Could you check a few things on this model? Use its own coordinates, in mm. Face numbers are marked on the shaded views. A direction names the side the tool comes from. Give positions to 0.01 mm unless a question says otherwise; leave off trailing zeros. Loops run counter-clockwise (first coordinate to the right, second up) from the corner with the lowest first, then second, coordinate; pieces in that order, holes last. Notation, with made-up numbers: (60, 72) - (102, 72) arc R14 ccw to (102, 86) - close; hole circle Ø1 at (72.5, 88). An arc over 180 degrees is marked (long way). One line per item, written item: value. Start each with the question number.
Q1. I want a section at D-D (z = -25). Please give me the cut outline in (x, y).
Q2. I want a section at C-C (z = 54.5). Please give me the cut outline in (x, y).
Q3. I want a section at A-A (z = 0). Please give me the cut outline in (x, y), then the cut area to 3 significant figures.
Q4. I want a section at B-B (y = -16). Please give me the cut outline in (x, z), then the cut area to 3 significant figures.
Q5. If I drill on line 1 (Y direction, x = 12, z = -1); line 2 (Y direction, x = 4, z = 43); line 3 (Z direction, x = -0.5, y = -39.5), over which ranges is the centre line in solid material (lowest first)? Write a range as from..to.
Q6. I'm going to push flat-ended pins straight in: P1, Ø1, axis at y = -1, z = -20.5, coming from the +X side; P2, Ø8, axis at x = 25.5, z = -15, coming from the -Y side; P3, Ø2, axis at x = 10, y = -43, coming from the +Z side; P4, Ø5, axis at x = 8, z = -6.5, coming from the +Y side. Where does each tip first touch, or does it pass through?
Q7. For the marked faces 5 and 6, which set-ups out of +Z, -Z, +X, -X, +Y, -Y let a thin tool reach every point of the face, with its end or its side?
Q8. If we mould it in two halves opening along Z, with no side actions, what happens to the marked faces 1, 2, 3 and 4? For each: released by +Z, released by -Z, zero draft, split by the parting line, or undercut.
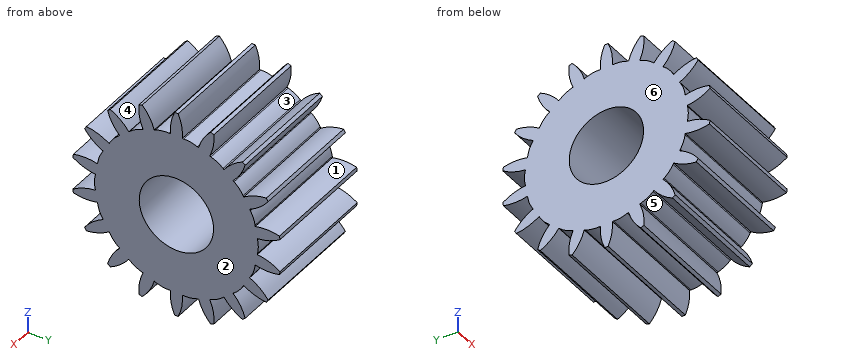
```python
from build123d import *

# Parameters (mm, degrees)
SKETCH1_R                = 63.5
BOSS_EXTRUDE1_DEPTH      = 35
SKETCH6_R                = 22.5
CUT_EXTRUDE4_DEPTH       = 71
CUT_EXTRUDE5_DEPTH       = 71
FILLET1_R                = 20
CIRPATTERN3_COUNT        = 18
FILLET1_OF_CIRPATTERN3_R = 20


with BuildPart() as part:
    # Sketch1 → Boss-Extrude1 (new body, symmetric)
    with BuildSketch(Plane(origin=(0, 0, 0), x_dir=(0, 0, -1), z_dir=(1, 0, 0))):
        Circle(SKETCH1_R)
    extrude(amount=BOSS_EXTRUDE1_DEPTH, both=True)

    # Sketch6 → Cut-Extrude4 (cut, through all)
    with BuildSketch(Plane(origin=(35, 0, 0), x_dir=(0, 0, -1), z_dir=(1, 0, 0))):
        Circle(SKETCH6_R)
    extrude(amount=-CUT_EXTRUDE4_DEPTH, mode=Mode.SUBTRACT)

    # Sketch7 → Cut-Extrude5 (cut, through all)
    with BuildSketch(Plane(origin=(35, 0, 0), x_dir=(0, 0, -1), z_dir=(1, 0, 0))):
        with BuildLine():
            Line((0, 50.039601818), (-4.985, 48.961883134))
            ThreePointArc((-4.985, 48.961883134), (-6.597219376, 56.157134763), (-9.975, 62.711636679))
            Line((-9.975, 62.711636679), (0, 72.167588378))
            Line((0, 72.167588378), (9.975, 62.711636679))
            ThreePointArc((9.975, 62.711636679), (6.597219376, 56.157134763), (4.985, 48.961883134))
            Line((4.985, 48.961883134), (0, 50.039601818))
        make_face()
    cut_extrude5 = extrude(amount=-CUT_EXTRUDE5_DEPTH, mode=Mode.SUBTRACT)

    # Fillet1
    fillet1_edges = [part.edges().sort_by_distance(p)[0] for p in [
        (0, 50.039601818, 0),
    ]]
    fillet(fillet1_edges, radius=FILLET1_R)

    # CirPattern3: Cut-Extrude5 ×18 about axis
    cirpattern3_axis = Axis((0, 0, 0), (1, 0, 0))
    for i in range(1, CIRPATTERN3_COUNT):
        add(cut_extrude5.rotate(cirpattern3_axis, i * 360 / CIRPATTERN3_COUNT), mode=Mode.SUBTRACT)

    # Fillet1 of CirPattern3
    fillet1_of_cirpattern3_edges = [part.edges().sort_by_distance(p)[0] for p in [
        (0, 47.021844575, 17.114551786),
        (0, 38.332558908, 32.164836042),
        (0, 25.019800909, 43.335566369),
        (0, 8.689285667, 49.279387828),
        (0, -8.689285667, 49.279387828),
        (0, -25.019800909, 43.335566369),
        (0, -38.332558908, 32.164836042),
        (0, -47.021844575, 17.114551786),
        (0, -50.039601818, 0),
        (0, -47.021844575, -17.114551786),
        (0, -38.332558908, -32.164836042),
        (0, -25.019800909, -43.335566369),
        (0, -8.689285667, -49.279387828),
        (0, 8.689285667, -49.279387828),
        (0, 25.019800909, -43.335566369),
        (0, 38.332558908, -32.164836042),
        (0, 47.021844575, -17.114551786),
    ]]
    fillet(fillet1_of_cirpattern3_edges, radius=FILLET1_OF_CIRPATTERN3_R)


solid = part.part
```
Worked answers:
1. outline: (-35, -50.02) - (35, -50.02) - (35, 50.02) - (-35, 50.02) - close
2. outline: (-35, -22.7) - (35, -22.7) - (35, -16.45) - (-35, -16.45) - close; (-35, -3.53) - (35, -3.53) - (35, 3.53) - (-35, 3.53) - close; (-35, 16.45) - (35, 16.45) - (35, 22.7) - (-35, 22.7) - close
3. outline: (-35, -49.58) - (35, -49.58) - (35, -22.5) - (-35, -22.5) - close; (-35, 22.5) - (35, 22.5) - (35, 49.58) - (-35, 49.58) - close
3. area: 3,790 mm²
4. outline: (-35, -53.72) - (35, -53.72) - (35, -15.82) - (-35, -15.82) - close; (-35, 15.82) - (35, 15.82) - (35, 53.72) - (-35, 53.72) - close
4. area: 5,310 mm²
5. line 1: y = -49.55..-22.48, 22.48..49.55
5. line 2: y = -39.76..-31.32, -24.68..24.68, 31.32..39.76
5. line 3: z = -49.08..-42.48, -29.8..29.8, 42.48..49.08
6. P1: passes through
6. P2: stops at y = -62.54
6. P3: stops at z = 29.62
6. P4: stops at y = 61.2
7. face 5: +X, -X
7. face 6: +Z, -Z, -X, +Y, -Y
8. face 1: undercut
8. face 2: zero draft
8. face 3: undercut
8. face 4: released by +Z
